```python
from build123d import *

# Parameters (mm, degrees)
SKETCH1_W               = 93
SKETCH1_H               = 65
SKETCH1_W_2             = 83
SKETCH1_H_2             = 55
BOSS_EXTRUDE1_DEPTH     = 8
FILLET1_R               = 3
SKETCH2_W               = 10
SKETCH2_H               = 4
BOSS_EXTRUDE6_DEPTH     = 8
FILLET3_R               = 3
SKETCH9_R               = 1.47
CUT_EXTRUDE1_DEPTH      = 5
MIRROR4_COPY_1_SKETCH_R = 1.47
MIRROR4_COPY_1_DEPTH    = 5
FILLET4_R               = 3
SKETCH10_W              = 2
SKETCH10_H              = 1
SKETCH10_W_2            = 5
CUT_EXTRUDE2_DEPTH      = 9
SKETCH11_W              = 2
SKETCH11_H              = 1
SKETCH11_W_2            = 5
CUT_EXTRUDE3_DEPTH      = 9
SKETCH12_W              = 1
SKETCH12_H              = 2
CUT_EXTRUDE4_DEPTH      = 9
SKETCH14_W              = 4
SKETCH14_H              = 2
BOSS_EXTRUDE14_DEPTH    = 4
SKETCH15_W              = 3.95
SKETCH15_H              = 2
BOSS_EXTRUDE18_DEPTH    = 6
SKETCH16_W              = 2
SKETCH16_H              = 4
SKETCH16_W_2            = 5
BOSS_EXTRUDE19_DEPTH    = 4
SKETCH17_W              = 2
SKETCH17_H              = 3.95
SKETCH17_W_2            = 5
BOSS_EXTRUDE20_DEPTH    = 6
SKETCH18_W              = 5
SKETCH18_H              = 3.95
SKETCH18_W_2            = 2
BOSS_EXTRUDE21_DEPTH    = 6
FILLET6_R               = 3


with BuildPart() as part:
    # Sketch1 → Boss-Extrude1 (new body)
    with BuildSketch(Plane.XY):
        Rectangle(SKETCH1_W, SKETCH1_H)
        Rectangle(SKETCH1_W_2, SKETCH1_H_2, mode=Mode.SUBTRACT)
    extrude(amount=BOSS_EXTRUDE1_DEPTH)

    # Fillet1
    fillet1_edges = [part.edges().sort_by_distance(p)[0] for p in [
        (-46.5, 32.5, 4),
        (46.5, 32.5, 4),
        (46.5, -32.5, 4),
        (-46.5, -32.5, 4),
    ]]
    fillet(fillet1_edges, radius=FILLET1_R)

    # Sketch2 → Boss-Extrude6 (add)
    with BuildSketch(Plane(origin=(0, 32.5, 0), x_dir=(1, 0, 0), z_dir=(0, 1, 0))):
        with Locations((-27.5, -2)):
            Rectangle(SKETCH2_W, SKETCH2_H)
        with Locations((27.5, -2)):
            Rectangle(SKETCH2_W, SKETCH2_H)
    boss_extrude6 = extrude(amount=BOSS_EXTRUDE6_DEPTH)

    # Mirror2: Boss-Extrude6 across plane
    add(boss_extrude6.mirror(Plane.ZX))

    # Fillet3
    fillet3_edges = [part.edges().sort_by_distance(p)[0] for p in [
        (32.5, -32.5, 2),
        (22.5, -32.5, 2),
        (-22.5, 32.5, 2),
        (-32.5, 32.5, 2),
        (32.5, 32.5, 2),
        (22.5, 32.5, 2),
        (-22.5, -32.5, 2),
        (-32.5, -32.5, 2),
    ]]
    fillet(fillet3_edges, radius=FILLET3_R)

    # Sketch9 → Cut-Extrude1 (cut, through all)
    with BuildSketch(Plane.XY.offset(4)):
        with Locations((27.5, -36.742693553)):
            Circle(SKETCH9_R)
    cut_extrude1 = extrude(amount=-CUT_EXTRUDE1_DEPTH, mode=Mode.SUBTRACT)

    # Mirror3: Cut-Extrude1 across plane
    add(cut_extrude1.mirror(Plane(origin=(0, 0, 0), x_dir=(0, 0, 1), z_dir=(1, 0, 0))), mode=Mode.SUBTRACT)

    # Mirror4: Cut-Extrude1 across plane
    add(cut_extrude1.mirror(Plane.ZX), mode=Mode.SUBTRACT)

    # Mirror4 copy 1 sketch → Mirror4 copy 1 (cut, through all)
    with BuildSketch(Plane(origin=(0, 0, 4), x_dir=(-1, 0, 0), z_dir=(0, 0, 1))):
        with Locations((27.5, -36.742693553)):
            Circle(MIRROR4_COPY_1_SKETCH_R)
    extrude(amount=-MIRROR4_COPY_1_DEPTH, mode=Mode.SUBTRACT)

    # Fillet4
    fillet4_edges = [part.edges().sort_by_distance(p)[0] for p in [
        (32.5, -40.5, 2),
        (22.5, -40.5, 2),
        (-22.5, 40.5, 2),
        (-32.5, 40.5, 2),
        (32.5, 40.5, 2),
        (22.5, 40.5, 2),
        (-22.5, -40.5, 2),
        (-32.5, -40.5, 2),
    ]]
    fillet(fillet4_edges, radius=FILLET4_R)

    # Sketch10 → Cut-Extrude2 (cut, through all)
    with BuildSketch(Plane(origin=(0, 0, 0), x_dir=(-1, 0, 0), z_dir=(0, 0, -1))):
        with Locations((-25.5, -28)):
            Rectangle(SKETCH10_W, SKETCH10_H)
        with Locations((26, -28)):
            Rectangle(SKETCH10_W_2, SKETCH10_H)
    extrude(amount=-CUT_EXTRUDE2_DEPTH, mode=Mode.SUBTRACT)

    # Sketch11 → Cut-Extrude3 (cut, through all)
    with BuildSketch(Plane(origin=(0, 0, 0), x_dir=(-1, 0, 0), z_dir=(0, 0, -1))):
        with Locations((25.5, 28)):
            Rectangle(SKETCH11_W, SKETCH11_H)
        with Locations((-26, 28)):
            Rectangle(SKETCH11_W_2, SKETCH11_H)
    extrude(amount=-CUT_EXTRUDE3_DEPTH, mode=Mode.SUBTRACT)

    # Sketch12 → Cut-Extrude4 (cut, through all)
    with BuildSketch(Plane(origin=(0, 0, 0), x_dir=(-1, 0, 0), z_dir=(0, 0, -1))):
        with Locations((-42, 0)):
            Rectangle(SKETCH12_W, SKETCH12_H)
        with Locations((-42, -23.5)):
            Rectangle(SKETCH12_W, SKETCH12_H)
        with Locations((-42, 23.5)):
            Rectangle(SKETCH12_W, SKETCH12_H)
    cut_extrude4 = extrude(amount=-CUT_EXTRUDE4_DEPTH, mode=Mode.SUBTRACT)

    # Mirror5: Cut-Extrude4 across plane
    add(cut_extrude4.mirror(Plane(origin=(0, 0, 0), x_dir=(0, 0, 1), z_dir=(1, 0, 0))), mode=Mode.SUBTRACT)

    # Sketch14 → Boss-Extrude14 (add)
    with BuildSketch(Plane.XY.offset(8)):
        with Locations((44.5, 23.5)):
            Rectangle(SKETCH14_W, SKETCH14_H)
        with Locations((44.5, 0)):
            Rectangle(SKETCH14_W, SKETCH14_H)
        with Locations((44.5, -23.5)):
            Rectangle(SKETCH14_W, SKETCH14_H)
    boss_extrude14 = extrude(amount=BOSS_EXTRUDE14_DEPTH)

    # Mirror6: Boss-Extrude14 across plane
    add(boss_extrude14.mirror(Plane(origin=(0, 0, 0), x_dir=(0, 0, 1), z_dir=(1, 0, 0))))

    # Sketch15 → Boss-Extrude18 (add)
    with BuildSketch(Plane.ZY.offset(-42.5)):
        with Locations((10.025, 23.5)):
            Rectangle(SKETCH15_W, SKETCH15_H)
        with Locations((10.025, 0)):
            Rectangle(SKETCH15_W, SKETCH15_H)
        with Locations((10.025, -23.5)):
            Rectangle(SKETCH15_W, SKETCH15_H)
    boss_extrude18 = extrude(amount=BOSS_EXTRUDE18_DEPTH)

    # Mirror7: Boss-Extrude18 across plane
    add(boss_extrude18.mirror(Plane(origin=(0, 0, 0), x_dir=(0, 0, 1), z_dir=(1, 0, 0))))

    # Sketch16 → Boss-Extrude19 (add)
    with BuildSketch(Plane.XY.offset(8)):
        with Locations((-25.5, 30.5)):
            Rectangle(SKETCH16_W, SKETCH16_H)
        with Locations((26, 30.5)):
            Rectangle(SKETCH16_W_2, SKETCH16_H)
        with Locations((25.5, -30.5)):
            Rectangle(SKETCH16_W, SKETCH16_H)
        with Locations((-26, -30.5)):
            Rectangle(SKETCH16_W_2, SKETCH16_H)
    extrude(amount=BOSS_EXTRUDE19_DEPTH)

    # Sketch17 → Boss-Extrude20 (add)
    with BuildSketch(Plane.XZ.offset(-28.5)):
        with Locations((-25.5, 10.025)):
            Rectangle(SKETCH17_W, SKETCH17_H)
        with Locations((26, 10.025)):
            Rectangle(SKETCH17_W_2, SKETCH17_H)
    extrude(amount=BOSS_EXTRUDE20_DEPTH)

    # Sketch18 → Boss-Extrude21 (add)
    with BuildSketch(Plane(origin=(0, -28.5, 0), x_dir=(1, 0, 0), z_dir=(0, 1, 0))):
        with Locations((-26, -10.025)):
            Rectangle(SKETCH18_W, SKETCH18_H)
        with Locations((25.5, -10.025)):
            Rectangle(SKETCH18_W_2, SKETCH18_H)
    extrude(amount=BOSS_EXTRUDE21_DEPTH)

    # Fillet6
    fillet6_edges = [part.edges().sort_by_distance(p)[0] for p in [
        (-25.5, 32.5, 12),
        (-25.5, 22.5, 12),
        (-36.5, 23.5, 12),
        (-46.5, 23.5, 12),
        (-36.5, 0, 12),
        (-46.5, 0, 12),
        (-36.5, -23.5, 12),
        (-46.5, -23.5, 12),
        (-26, -32.5, 12),
        (-26, -22.5, 12),
        (25.5, -32.5, 12),
        (25.5, -22.5, 12),
        (36.5, -23.5, 12),
        (46.5, -23.5, 12),
        (46.5, 0, 12),
        (36.5, 0, 12),
        (36.5, 23.5, 12),
        (26, 22.5, 12),
        (26, 32.5, 12),
        (46.5, 23.5, 12),
    ]]
    fillet(fillet6_edges, radius=FILLET6_R)


solid = part.part
```
Model file for the job. Use its own axes, mm. A direction names the side the tool comes from. Round coordinates to 2 decimals unless told otherwise and drop trailing zeros. Order: outer loops, then holes, each group sorted by start corner. A loop starts at its lowest first (then second) coordinate and runs counter-clockwise, first axis right, second up. Notation, with made-up numbers: (-14.75, 27) -> (30.25, 27) arc R23 ccw to (30.25, 63) -> close; hole circle Ø4 at (85, 61). An arc over 180 degrees is marked (long way). Use one line per item in the form item = value.
Item 1: Cut at B-B, the plane y = -5. Write the cut outline in (x, z).
Returned:
outline = (-46.5, 0) -> (-41.5, 0) -> (-41.5, 8) -> (-46.5, 8) -> close; (41.5, 0) -> (46.5, 0) -> (46.5, 8) -> (41.5, 8) -> close
Item 2: Pull direction X, two halves, no side cores. Call faces 1 (the face through (40, -24, 8.05)), 2 (the face through (41, 1, 10)), 3 (the face through (-46.5, 0, 4)): released by +X, released by -X, zero draft, split by the parting line, or undercut.
Returned:
face_1 = undercut
face_2 = zero draft
face_3 = released by -X
Item 3: Drill centre lines: line 1 (Y direction, x = -27.5, z = 1.45); line 2 (Y direction, x = 27.5, z = 3.1); line 3 (X direction, y = 24, z = 9). Where is each one in solid material? Low to high.
Returned:
line_1 = -40.5 to -38.21, -35.27 to -28.5, 27.5 to 35.27, 38.21 to 40.5
line_2 = -40.5 to -38.21, -35.27 to -27.5, 28.5 to 35.27, 38.21 to 40.5
line_3 = -46.5 to -36.5, -26.5 to -24.5, 23.5 to 28.5, 36.5 to 46.5
Item 4: Cut at A-A, the plane x = 27.5. Write the cut outline in (y, z), and give its area (3 significant figures).
Returned:
outline = (-40.5, 0) -> (-38.21, 0) -> (-38.21, 4) -> (-40.5, 4) -> close; (-35.27, 0) -> (-27.5, 0) -> (-27.5, 8) -> (-32.5, 8) -> (-32.5, 4) -> (-35.27, 4) -> close; (22.5, 8.05) -> (28.5, 8.05) -> (28.5, 0) -> (35.27, 0) -> (35.27, 4) -> (32.5, 4) -> (32.5, 9) arc R3 ccw to (29.5, 12) -> (25.5, 12) arc R3 ccw to (22.5, 9) -> close; (38.21, 0) -> (40.5, 0) -> (40.5, 4) -> (38.21, 4) -> close
area = 148 mm^2
Item 5: Tool access for faces 4 (the face through (22.5, 36, 2)), 5 (the face through (-41.5, -26, 4)), 6 (the face through (-42.5, 23, 4)), 7 (the face through (-42, 22.5, 10)): list every direction of +Z, -Z, +X, -X, +Y, -Y with a clear straight run to the whole face (end or side of a thin tool).
Returned:
face_4 = +Z, -Z, +Y
face_5 = +Z, -Z
face_6 = -Z
face_7 = +Z, +X, -X
Item 6: Cut at C-C, the plane x = -16.5. Write the cut outline in (y, z), and give its area (3 significant figures).
Returned:
outline = (-32.5, 0) -> (-27.5, 0) -> (-27.5, 8) -> (-32.5, 8) -> close; (27.5, 0) -> (32.5, 0) -> (32.5, 8) -> (27.5, 8) -> close
area = 80.0 mm^2
Item 7: Flat gauge pins, fed straight in: pin 1 Ø2.5 at (x, z) = (34, 4) entering from -Y; pin 2 Ø1.1 at (x, z) = (-42, 2) entering from +Y; pin 3 Ø0.8 at (x, z) = (-42, 3) entering from -Y. Where does each tip first touch, or does it go through?
Returned:
pin_1 = -34.3
pin_2 = 32.5
pin_3 = -32.5
